Could you check a few things on this drawing? It's one solid part, dimensions in mm from its lowest x, y, z. Give positions to 0.01 mm unless a question says otherwise; leave off trailing zeros. Write each loop counter-clockwise with the first axis right and the second up, starting at its lowest first coordinate (ties: lowest second). Pieces come first, ordered by that corner, then holes. Notation, with made-up numbers: M 81,66 L 114,66 A19 ccw 114,74 Z; hole C 32,66.25 d11. An arc over 180 degrees is marked long. Write each question's results on one line, items separated by ' | '. Start each with the question number.
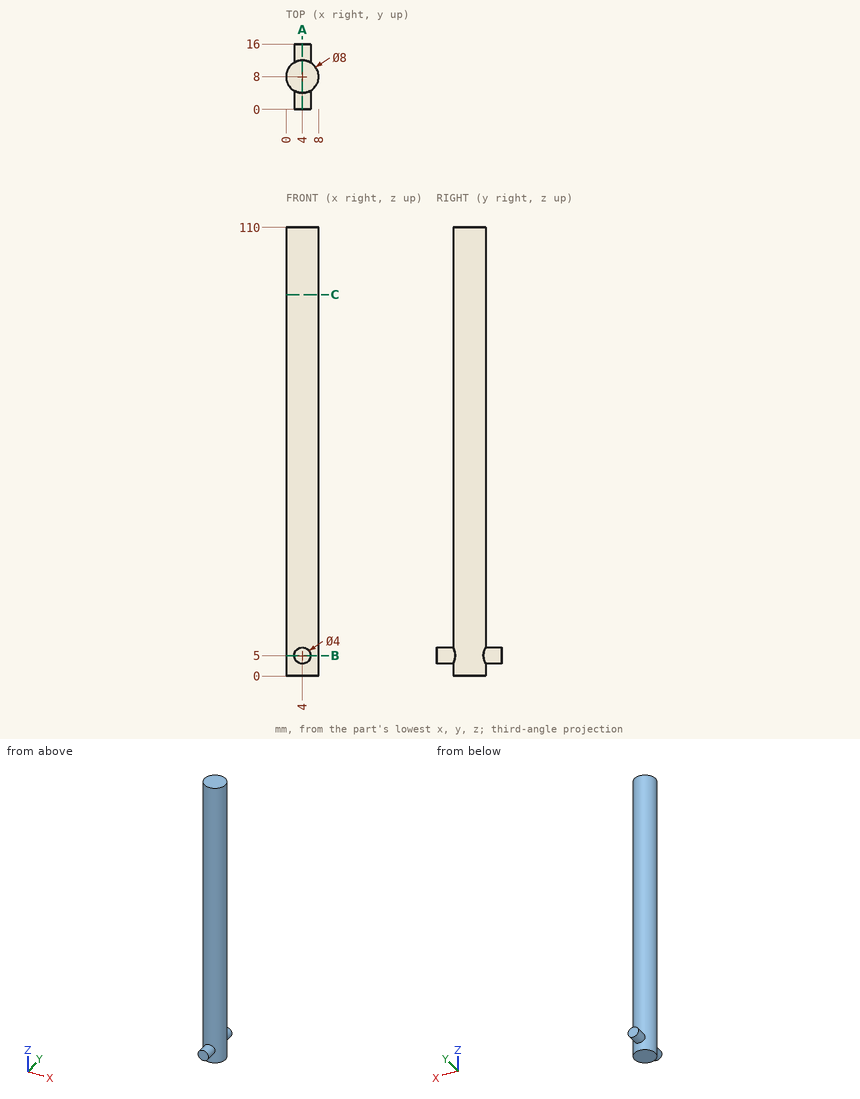
Q1. I'm going to push flat-ended pins straight in: P1, Ø4, axis at y = 3.5, z = 63.5, coming from the +X side; P2, Ø2, axis at y = 4, z = 40, coming from the +X side; P3, Ø1, axis at x = 7, y = 13, coming from the +Z side; P4, Ø1, axis at x = 3.5, z = 36.5, coming from the +Y side. Where does each tip first touch, or does it pass through?
Q2. If we section it at C-C (z = 93.5): Please give me the cut outline in (x, y).
Q3. If we section it at B-B (z = 5): Please give me the cut outline in (x, y), plus the area to 3 significant figures.
Q4. Please list where these lines run through material, in increasing order: line 1 (X direction, y = 8.25, z = 65.5); line 2 (Y direction, x = 4.25, z = 15); line 3 (X direction, y = 9.25, z = 7). Write a range as [from, to].
Q5. If we section it at A-A (x = 4): Please give me the cut outline in (y, z).
Determined:
1) P1: stops at x = 7.12 | P2: stops at x = 6.65 | P3: passes through | P4: stops at y = 12
2) outline: C 4,8 d8
3) outline: M 2,0 L 6,0 L 6,4.54 A4 ccw 6,11.46 L 6,16 L 2,16 L 2,11.46 A4 ccw 2,4.54 Z | area: 83.7 mm²
4) line 1: x = [0.01, 7.99] | line 2: y = [4.01, 11.99] | line 3: x = [0.2, 7.8]
5) outline: M 0,3 L 4,3 L 4,0 L 12,0 L 12,3 L 16,3 L 16,7 L 12,7 L 12,110 L 4,110 L 4,7 L 0,7 Z
